```python
from build123d import *

# Parameters (mm, degrees)
F0_W     = 203.2
F0_H     = 25.231637
F1_DEPTH = 25.4
F2_R     = 6.35
F3_DEPTH = 25.4
F5_DEPTH = 7.62
F6_R     = 25.4
F7_R     = 25.4


with BuildPart() as f1:
    # F0 (on Top) → F1 (new body)
    with BuildSketch(Plane.XY):
        with Locations((-101.6, 76.284181)):
            Rectangle(F0_W, F0_H)
        Polygon((0, 63.668363), (0, 0), (254, 0), (254, 152.4), (0, 152.4), (0, 88.9), align=None)
    extrude(amount=-F1_DEPTH)

    # F2 (on face) → F3 (cut)
    with BuildSketch(Plane.XY):
        with Locations((-190.5, 76.368363)):
            Circle(F2_R)
    extrude(amount=-F3_DEPTH, mode=Mode.SUBTRACT)

    # F4 (on face) → F5 (cut)
    with BuildSketch(Plane.XY):
        Polygon((241.3, 139.7), (12.7, 139.7), (12.7, 76.368363), (12.7, 76.2), (12.7, 12.7), (241.3, 12.7), align=None)
        Polygon((19.05, 82.718363), (19.05, 133.35), (234.95, 133.35), (234.95, 19.05), (19.05, 19.05), (19.05, 69.85), align=None, mode=Mode.SUBTRACT)
    extrude(amount=-F5_DEPTH, mode=Mode.SUBTRACT)

    # F6
    f6_edges = [f1.edges().sort_by_distance(p)[0] for p in [
        (0, 152.4, -12.7),
        (0, 88.9, -12.7),
    ]]
    fillet(f6_edges, radius=F6_R)

    # F7
    f7_edges = [f1.edges().sort_by_distance(p)[0] for p in [
        (0, 63.668363, -12.7),
        (0, 0, -12.7),
        (254, 152.4, -12.7),
        (254, 0, -12.7),
    ]]
    fillet(f7_edges, radius=F7_R)


solid = f1.part
```
Could you check a few things on this model? Use its own coordinates, in mm. A direction names the side the tool comes from. Coordinates: 2 decimals unless noted, no trailing zeros. Write each loop counter-clockwise with the first axis right and the second up, starting at its lowest first coordinate (ties: lowest second). Pieces come first, ordered by that corner, then holes. Notation, with made-up numbers: (46.25, 38.5) - (92.25, 38.5) arc R38 ccw to (92.25, 77.5) - close; hole circle Ø9 at (36.25, 40). An arc over 180 degrees is marked (long way). Use a Markdown table: item, result.
Q1. Imagine slicing it at C-C (z = -15.5). List the corners of the cut face in (x, y) for me.
Geometry check:
| item | result |
|---|---|
| outline | (-203.2, 63.67) - (-25.4, 63.67) arc R25.4 cw to (0, 38.27) - (0, 25.4) arc R25.4 ccw to (25.4, 0) - (228.6, 0) arc R25.4 ccw to (254, 25.4) - (254, 127) arc R25.4 ccw to (228.6, 152.4) - (25.4, 152.4) arc R25.4 ccw to (0, 127) - (0, 114.3) arc R25.4 cw to (-25.4, 88.9) - (-203.2, 88.9) - close; hole circle Ø12.7 at (-190.5, 76.37) |
Q2. Which directions (+Z, -Z, +X, -X, +Y, -Y) give clear straight access to the entire face, cutting with the end or side of a thin tool? Please do faces 1 (the cylindrical face through (246.36, 145.16, -12.88)), 2 (the flat face through (19.05, 75, -4)).
Geometry check:
| item | result |
|---|---|
| face 1 | +Z, -Z, +X, +Y |
| face 2 | +Z |
Q3. Imagine slicing it at A-A (x = -190.5). List the corners of the cut face in (y, z) for me, and give its area (3 significant figures).
Geometry check:
| item | result |
|---|---|
| outline | (63.67, -25.4) - (70.02, -25.4) - (70.02, 0) - (63.67, 0) - close; (82.72, -25.4) - (88.9, -25.4) - (88.9, 0) - (82.72, 0) - close |
| area | 318 mm2 |
Q4. Imagine slicing it at B-B (y = 30). List the corners of the cut face in (x, z) for me.
Geometry check:
| item | result |
|---|---|
| outline | (0, -25.4) - (254, -25.4) - (254, 0) - (241.3, 0) - (241.3, -7.62) - (234.95, -7.62) - (234.95, 0) - (19.05, 0) - (19.05, -7.62) - (12.7, -7.62) - (12.7, 0) - (0, 0) - close |
Q5. Imagine slicing it at D-D (x = 78.5). List the corners of the cut face in (y, z) for me.
Geometry check:
| item | result |
|---|---|
| outline | (0, -25.4) - (152.4, -25.4) - (152.4, 0) - (139.7, 0) - (139.7, -7.62) - (133.35, -7.62) - (133.35, 0) - (19.05, 0) - (19.05, -7.62) - (12.7, -7.62) - (12.7, 0) - (0, 0) - close |
Q6. I'm going to push flat-ended pins straight in: pin 1 Ø1.5 at (y, z) = (113, -19.5) entering from -X; pin 2 Ø7.5 at (x, z) = (-146.5, -16) entering from +Y; pin 3 Ø10 at (y, z) = (120.5, -17) entering from -X. Where does each tip first touch, or does it pass through?
Geometry check:
| item | result |
|---|---|
| pin 1 | stops at x = -0.08 |
| pin 2 | stops at y = 88.9 |
| pin 3 | stops at x = 0 |
Q7. Thinking about a two-plate mould opening in Y: for faces 3 (the flat face through (-203.2, 76, -13)), 4 (the flat face through (-116, 63.668, -13)), 5 (the flat face through (125, 12.7, -4)), 6 (the cylindrical face through (-7.64, 96.14, -12.88)), which applies, +Y half, -Y half, draft (parallel to the pull), parting line (faces both ways), or undercut?
Geometry check:
| item | result |
|---|---|
| face 3 | draft |
| face 4 | -Y half |
| face 5 | undercut |
| face 6 | +Y half |
Q8. Please list where these lines run through material, in increasing order: L1, parallel to Y at x = 179, z = -7.5; L2, parallel to X at y = 27.5, z = -6; L3, parallel to Y at x = -190.5, z = -13.5.
Geometry check:
| item | result |
|---|---|
| L1 | y = 0 to 12.7, 19.05 to 133.35, 139.7 to 152.4 |
| L2 | x = 0 to 12.7, 19.05 to 234.95, 241.3 to 254 |
| L3 | y = 63.67 to 70.02, 82.72 to 88.9 |
